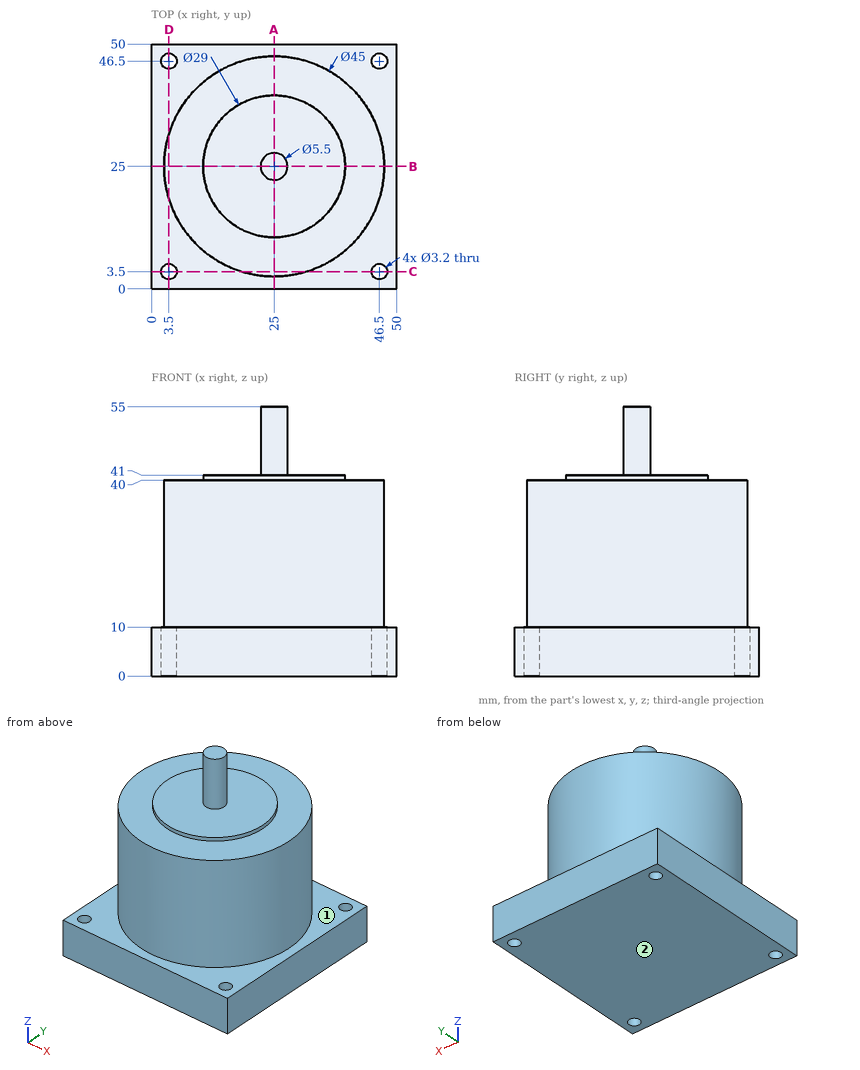
Study the drawing (mm; zero at the part's minimum x, y, z) and answer. A direction names the side the tool comes from. Coordinates: 2 decimals unless noted, no trailing zeros. Loops run counter-clockwise (first coordinate to the right, second up) from the corner with the lowest first, then second, coordinate; pieces in that order, holes last. Notation, with made-up numbers: M -19.75,68 L 37.25,68 A13 ccw 37.25,88 Z; hole C 3,24 d7. An arc over 180 degrees is marked long. Answer as a JSON object with one key per item and string values. Group by question number.
Item 1: Consider L1, parallel to Y at x = 3.5, z = 6.25; L2, parallel to Z at x = 43, y = 8; L3, parallel to Z at x = 30.5, y = 10. Determine where each line is inside the solid, lowest interval first.
Item 2: Each of these flat-tipped pins is pushed along its axis until it touches: P1, Ø5, axis at x = 34, y = 12, coming from the +Z side; P2, Ø4, axis at x = 5.5, z = 28, coming from the +Y side; P3, Ø4, axis at x = 3.5, y = 46.5, coming from the +Z side. Where does it stop, or does it pass through?
Item 3: Which of the six approach directions +Z, -Z, +X, -X, +Y, -Y give full straight-line access (tool end or side, diameter ignored) to the marked faces 1 and 2?
Item 4: Section C-C (y = 3.5) is taken. Write down the section's boundary in (x, z).
Item 5: Section A-A (x = 25) is taken. Write down the section's boundary in (y, z), and give its area (3 significant figures).
Solved:
{
 "1": {"L1": "y = 0 to 1.9, 5.1 to 44.9, 48.1 to 50", "L2": "z = 0 to 10", "L3": "z = 0 to 40"},
 "2": {"P1": "stops at z = 41", "P2": "stops at y = 39.14", "P3": "stops at z = 10"},
 "3": {"face 1": "+Z", "face 2": "-Z, +X, -X, +Y, -Y"},
 "4": {"outline": "M 0,0 L 1.9,0 L 1.9,10 L 0,10 Z; M 5.1,0 L 44.9,0 L 44.9,10 L 31.63,10 L 31.63,40 L 18.37,40 L 18.37,10 L 5.1,10 Z; M 48.1,0 L 50,0 L 50,10 L 48.1,10 Z"},
 "5": {"outline": "M 0,0 L 50,0 L 50,10 L 47.5,10 L 47.5,40 L 39.5,40 L 39.5,41 L 27.75,41 L 27.75,55 L 22.25,55 L 22.25,41 L 10.5,41 L 10.5,40 L 2.5,40 L 2.5,10 L 0,10 Z", "area": "1,960 mm2"}
}
